Could you check a few things on this drawing? It's one solid part, dimensions in mm from its lowest x, y, z. Round coordinates to 2 decimals unless told otherwise and drop trailing zeros. Order: outer loops, then holes, each group sorted by start corner. A loop starts at its lowest first (then second) coordinate and runs counter-clockwise, first axis right, second up. Notation, with made-up numbers: M 17,51 L 34,51 A30 ccw 34,84 Z; hole C 30,-13.75 d6. An arc over 180 degrees is marked long. Answer as a JSON object with one key per item and string values. Group by question number.
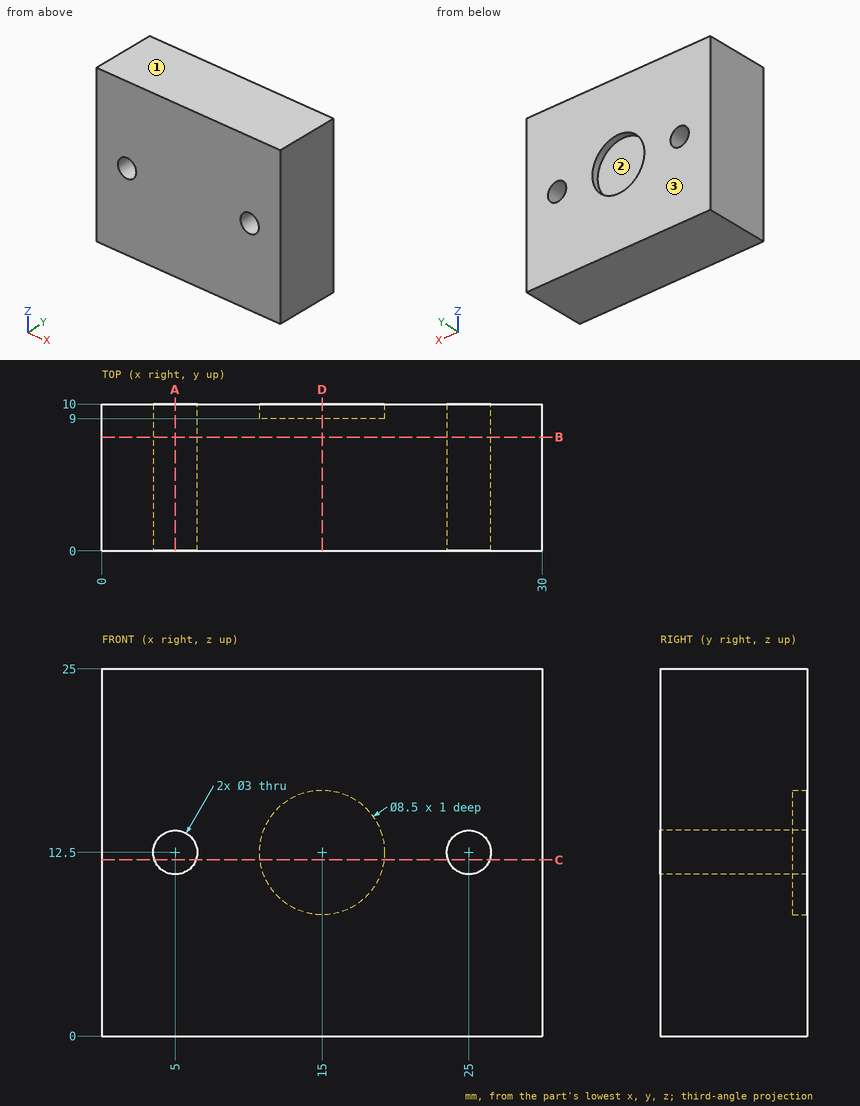
1) I need wall thicknesses on line 1 along X through (y, z) = (6.25, 12.5); line 2 along X through (y, z) = (9.35, 12.5); line 3 along X through (y, z) = (1.5, 13.5). Which ranges of each line are inside material? Lowest first, please.
2) If we section it at B-B on y = 7.75: Write out the boundary of the cut face in (x, z).
3) We'd pull the mould along Z, two halves only. Please class the marked faces 1, 2 and 3: +Z half, -Z half, draft (parallel to the pull), parting line (faces both ways), or undercut.
4) If we section it at C-C on z = 12: Write out the boundary of the cut face in (x, y).
5) For pin 1 (7.5 mm diameter, centred on x = 15, z = 12.5, fed in from -Y); pin 2 (2.5 mm diameter, centred on x = 14, z = 13, fed in from +Y), each with a flat end and sliding along its axis, tell me the tip position at first contact or that it passes through.
6) If we section it at A-A on x = 5: Write out the boundary of the cut face in (y, z), plus the area to 3 significant figures.
7) If we section it at D-D on x = 15: Write out the boundary of the cut face in (y, z).
Findings:
{
 "1": {"line 1": "x = 0 to 3.5, 6.5 to 23.5, 26.5 to 30", "line 2": "x = 0 to 3.5, 6.5 to 10.75, 19.25 to 23.5, 26.5 to 30", "line 3": "x = 0 to 3.88, 6.12 to 23.88, 26.12 to 30"},
 "2": {"outline": "M 0,0 L 30,0 L 30,25 L 0,25 Z; hole C 5,12.5 d3; hole C 25,12.5 d3"},
 "3": {"face 1": "+Z half", "face 2": "undercut", "face 3": "draft"},
 "4": {"outline": "M 0,0 L 3.59,0 L 3.59,10 L 0,10 Z; M 6.41,0 L 23.59,0 L 23.59,10 L 19.22,10 L 19.22,9 L 10.78,9 L 10.78,10 L 6.41,10 Z; M 26.41,0 L 30,0 L 30,10 L 26.41,10 Z"},
 "5": {"pin 1": "stops at y = 0", "pin 2": "stops at y = 9"},
 "6": {"outline": "M 0,0 L 10,0 L 10,11 L 0,11 Z; M 0,14 L 10,14 L 10,25 L 0,25 Z", "area": "220 mm^2"},
 "7": {"outline": "M 0,0 L 10,0 L 10,8.25 L 9,8.25 L 9,16.75 L 10,16.75 L 10,25 L 0,25 Z"}
}
